```python
from build123d import *

# Parameters (mm, degrees)
F0_W     = 105
F0_H     = 60
F1_DEPTH = 20
F2_R     = 7.5
F3_DEPTH = 15
F4_R     = 2.5


with BuildPart() as f1:
    # F0 (on Front) → F1 (new body)
    with BuildSketch(Plane.XZ):
        Rectangle(F0_W, F0_H)
    extrude(amount=F1_DEPTH)

    # F2 (on face) → F3 (cut)
    with BuildSketch(Plane.XZ.offset(20)):
        with BuildLine():
            ThreePointArc((-7.5, 0), (0, -7.5), (7.5, 0))
            ThreePointArc((7.5, 0), (0, 7.5), (-7.5, 0))
        make_face()
        with Locations((-25, 0)):
            Circle(F2_R)
        with BuildLine():
            ThreePointArc((32.5, 0), (25, 7.5), (17.5, 0))
            ThreePointArc((17.5, 0), (25, -7.5), (32.5, 0))
        make_face()
    extrude(amount=-F3_DEPTH, mode=Mode.SUBTRACT)

    # F4
    f4_edges = [f1.edges().sort_by_distance(p)[0] for p in [
        (-52.5, -20, 0),
        (0, -20, -30),
        (52.5, -20, 0),
        (0, -20, 30),
        (-52.5, 0, 0),
        (0, 0, 30),
        (52.5, 0, 0),
        (0, 0, -30),
    ]]
    fillet(f4_edges, radius=F4_R)


solid = f1.part
```
Source: CAD feature listing. Evaluate the final solid. Frame: model axes, mm. A direction names the side the tool comes from. Give positions to 0.01 mm unless a question says otherwise; leave off trailing zeros. Loops run counter-clockwise (first coordinate to the right, second up) from the corner with the lowest first, then second, coordinate; pieces in that order, holes last. Notation, with made-up numbers: (50, -37) - (109, -37) arc R18 ccw to (109, -18) - close; hole circle Ø3 at (26, 24.25). An arc over 180 degrees is marked (long way). Use CSV: the item, a comma, the result in double quotes.
1) Line query: line 1 (Z direction, x = 0, y = -12); line 2 (X direction, y = -17.75, z = -4); line 3 (X direction, y = -10.25, z = 1). Output: solid intervals per line, ascending.
Worked out:
line 1,"z = -30 to -7.5, 7.5 to 30"
line 2,"x = -52.49 to -31.34, -18.66 to -6.34, 6.34 to 18.66, 31.34 to 52.49"
line 3,"x = -52.5 to -32.43, -17.57 to -7.43, 7.43 to 17.57, 32.43 to 52.5"
2) Cut plane A-A (z = 0). Output: boundary loops of the cut face in (x, y), and give its area (3 significant figures).
Worked out:
outline,"(-52.5, -17.5) arc R2.5 ccw to (-50, -20) - (-32.5, -20) - (-32.5, -5) - (-17.5, -5) - (-17.5, -20) - (-7.5, -20) - (-7.5, -5) - (7.5, -5) - (7.5, -20) - (17.5, -20) - (17.5, -5) - (32.5, -5) - (32.5, -20) - (50, -20) arc R2.5 ccw to (52.5, -17.5) - (52.5, -2.5) arc R2.5 ccw to (50, 0) - (-50, 0) arc R2.5 ccw to (-52.5, -2.5) - close"
area,"1,420 mm^2"
3) Pin query (flat end, axial travel): P1, Ø7.5, axis at x = 28, z = -2, coming from the -Y side. Return the tip coordinate at first contact, or that it passes through.
Worked out:
P1,"stops at y = -5"
4) Mould query, pull axis X, two halves, no side actions, for faces 1 (the cylindrical face through (0.735, -19.248, 29.287)), 2 (the flat face through (25, -5, 0)), 3 (the cylindrical face through (-52, -19, 0)). Classes: +X half, -X half, draft (parallel to the pull), parting line (faces both ways), or undercut.
Worked out:
face 1,"draft"
face 2,"undercut"
face 3,"-X half"
5) Set-up query: faces 4 (the cylindrical face through (-32.493, -12.605, 0.33)), 5 (the cylindrical face through (52, -1, 0)). Return all of +Z, -Z, +X, -X, +Y, -Y with unobstructed straight access to the full face (end or side cutting, diameter ignored); none if empty.
Worked out:
face 4,"-Y"
face 5,"+Z, -Z, +X, +Y"
6) Cut plane B-B (x = 0). Output: boundary loops of the cut face in (y, z), and give its area (3 significant figures).
Worked out:
outline,"(-20, -27.5) arc R2.5 ccw to (-17.5, -30) - (-2.5, -30) arc R2.5 ccw to (0, -27.5) - (0, 27.5) arc R2.5 ccw to (-2.5, 30) - (-17.5, 30) arc R2.5 ccw to (-20, 27.5) - (-20, 7.5) - (-5, 7.5) - (-5, -7.5) - (-20, -7.5) - close"
area,"970 mm^2"
